```python
from build123d import *

# Parameters (mm, degrees)
F0_W      = 120.65
F0_H      = 120.65
F1_DEPTH  = 1.5875
F2_W      = 12.7
F2_H      = 6.35
F3_DEPTH  = 1.5875
F4_W      = 12.7
F4_H      = 6.35
F5_DEPTH  = 1.5875
F6_W      = 6.35
F6_H      = 6.35
F7_DEPTH  = 1.5875
F8_W      = 12.7
F8_H      = 6.35
F9_DEPTH  = 1.5875
F10_W     = 12.7
F10_H     = 6.35
F11_DEPTH = 1.5875
F12_W     = 6.35
F12_H     = 12.7
F13_DEPTH = 1.5875
F14_W     = 6.35
F14_H     = 12.7
F15_DEPTH = 1.5875
F16_W     = 6.35
F16_H     = 12.7
F17_DEPTH = 1.5875
F18_W     = 12.7
F18_H     = 6.35
F19_DEPTH = 1.5875
F20_W     = 12.7
F20_H     = 6.35
F20_W_2   = 6.35
F21_DEPTH = 1.5875
F22_W     = 6.35
F22_H     = 12.7
F23_DEPTH = 1.5875
F24_W     = 6.35
F24_H     = 12.7
F25_DEPTH = 1.5875


with BuildPart() as f1:
    # F0 (on Right) → F1 (new body)
    with BuildSketch(Plane.YZ):
        Rectangle(F0_W, F0_H)
    extrude(amount=F1_DEPTH)

    # F2 (on face) → F3 (cut)
    with BuildSketch(Plane(origin=(0, 0, 0), x_dir=(0, -1, 0), z_dir=(-1, 0, 0))):
        with Locations((53.975, 57.15)):
            Rectangle(F2_W, F2_H)
    extrude(amount=-F3_DEPTH, mode=Mode.SUBTRACT)

    # F4 (on face) → F5 (cut)
    with BuildSketch(Plane(origin=(0, 0, 0), x_dir=(0, -1, 0), z_dir=(-1, 0, 0))):
        with Locations((28.575, 57.15)):
            Rectangle(F4_W, F4_H)
    extrude(amount=-F5_DEPTH, mode=Mode.SUBTRACT)

    # F6 (on face) → F7 (cut)
    with BuildSketch(Plane(origin=(0, 0, 0), x_dir=(0, -1, 0), z_dir=(-1, 0, 0))):
        with Locations((0, 57.15)):
            Rectangle(F6_W, F6_H)
    extrude(amount=-F7_DEPTH, mode=Mode.SUBTRACT)

    # F8 (on face) → F9 (cut)
    with BuildSketch(Plane(origin=(0, 0, 0), x_dir=(0, -1, 0), z_dir=(-1, 0, 0))):
        with Locations((-53.975, 57.15)):
            Rectangle(F8_W, F8_H)
    extrude(amount=-F9_DEPTH, mode=Mode.SUBTRACT)

    # F10 (on face) → F11 (cut)
    with BuildSketch(Plane(origin=(0, 0, 0), x_dir=(0, -1, 0), z_dir=(-1, 0, 0))):
        with Locations((-28.575, 57.15)):
            Rectangle(F10_W, F10_H)
    extrude(amount=-F11_DEPTH, mode=Mode.SUBTRACT)

    # F12 (on face) → F13 (cut)
    with BuildSketch(Plane(origin=(0, 0, 0), x_dir=(0, -1, 0), z_dir=(-1, 0, 0))):
        with Locations((-57.15, 34.925)):
            Rectangle(F12_W, F12_H)
    extrude(amount=-F13_DEPTH, mode=Mode.SUBTRACT)

    # F14 (on face) → F15 (cut)
    with BuildSketch(Plane(origin=(0, 0, 0), x_dir=(0, -1, 0), z_dir=(-1, 0, 0))):
        with Locations((-57.15, 4.7625)):
            Rectangle(F14_W, F14_H)
    extrude(amount=-F15_DEPTH, mode=Mode.SUBTRACT)

    # F16 (on face) → F17 (cut)
    with BuildSketch(Plane(origin=(0, 0, 0), x_dir=(0, -1, 0), z_dir=(-1, 0, 0))):
        with Locations((-57.15, -25.4)):
            Rectangle(F16_W, F16_H)
    extrude(amount=-F17_DEPTH, mode=Mode.SUBTRACT)

    # F18 (on face) → F19 (cut)
    with BuildSketch(Plane(origin=(0, 0, 0), x_dir=(0, -1, 0), z_dir=(-1, 0, 0))):
        with Locations((-53.975, -57.15)):
            Rectangle(F18_W, F18_H)
        with Locations((53.975, -57.15)):
            Rectangle(F18_W, F18_H)
    extrude(amount=-F19_DEPTH, mode=Mode.SUBTRACT)

    # F20 (on face) → F21 (cut)
    with BuildSketch(Plane(origin=(0, 0, 0), x_dir=(0, -1, 0), z_dir=(-1, 0, 0))):
        with Locations((-28.575, -57.15)):
            Rectangle(F20_W, F20_H)
        with Locations((0, -57.15)):
            Rectangle(F20_W_2, F20_H)
        with Locations((28.575, -57.15)):
            Rectangle(F20_W, F20_H)
    extrude(amount=-F21_DEPTH, mode=Mode.SUBTRACT)

    # F22 (on face) → F23 (cut)
    with BuildSketch(Plane(origin=(0, 0, 0), x_dir=(0, -1, 0), z_dir=(-1, 0, 0))):
        with Locations((57.15, 34.925)):
            Rectangle(F22_W, F22_H)
        with Locations((57.15, 4.7625)):
            Rectangle(F22_W, F22_H)
    extrude(amount=-F23_DEPTH, mode=Mode.SUBTRACT)

    # F24 (on face) → F25 (cut)
    with BuildSketch(Plane(origin=(0, 0, 0), x_dir=(0, -1, 0), z_dir=(-1, 0, 0))):
        with Locations((57.15, -25.4)):
            Rectangle(F24_W, F24_H)
    extrude(amount=-F25_DEPTH, mode=Mode.SUBTRACT)


solid = f1.part
```
The model under review builds one solid part; all positions refer to its coordinate system, in mm. Round coordinates to 2 decimals unless told otherwise and drop trailing zeros. Loops run counter-clockwise (first coordinate to the right, second up) from the corner with the lowest first, then second, coordinate; pieces in that order, holes last. Notation, with made-up numbers: (63.5, 31.5) -> (107.5, 31.5) arc R24 cw to (107.5, 67.5) -> close; hole circle Ø3 at (-30.75, 28.5). An arc over 180 degrees is marked (long way). Answer in a Markdown table with one row per item.
1) For pin 1 Ø0.8 at (x, y) = (0.5, 56) entering from +Z (3 decimals); pin 2 Ø0.8 at (x, z) = (0.5, -56) entering from -Y (3 decimals); pin 3 Ø0.8 at (x, z) = (0.5, 3.5) entering from +Y (3 decimals), all flat-tipped, find the tip position at first contact; note any pin that passes through.
Taken from the geometry:
| item | result |
|---|---|
| pin 1 | stops at z = 53.975 |
| pin 2 | stops at y = -47.625 |
| pin 3 | stops at y = 53.975 |
2) Consider section A-A, the plane z = -21. Write out the cut boundary in (x, y) (1 decimal), plus the area to 3 significant figures.
Taken from the geometry:
| item | result |
|---|---|
| outline | (0, -54) -> (1.6, -54) -> (1.6, 54) -> (0, 54) -> close |
| area | 171 mm² |
3) Wall thickness on line 1 along Z through (x, y) = (0.8, -33.5) (3 decimals): over which ranges is the line inside the solid? List them lowest first.
Taken from the geometry:
| item | result |
|---|---|
| line 1 | z = -53.975 to 53.975 |
